from build123d import *

# Parameters (mm, degrees)
RESSALTO_EXTRUS_O1_DEPTH = 2
ESBO_O3_R                = 2
CORTE_EXTRUS_O2_DEPTH    = 10
ESBO_O5_R                = 1.65
CORTE_EXTRUS_O5_DEPTH    = 2


with BuildPart() as part:
    # Esboço1 → Ressalto-extrusão1 (new body)
    with BuildSketch(Plane(origin=(0, 0, 0), x_dir=(1, 0, 0), z_dir=(0, 1, 0))):
        Polygon((-114, 41.685), (-114, -79.875), (-51, -79.875), (0, -79.875), (0, 79.875), (-69.415, 79.875), align=None)
        Polygon((0, 79.875), (0, -79.875), (51.996049983, -79.875), (114, -79.875), (114, 41.685), (69.415, 79.875), align=None)
    extrude(amount=RESSALTO_EXTRUS_O1_DEPTH)

    # Esboço3 → Corte-extrusão2 (cut)
    with BuildSketch(Plane(origin=(0, 2, 0), x_dir=(1, 0, 0), z_dir=(0, 1, 0))):
        with Locations(Location((-45.14, -69.875, 0), (0, 0, 270))):
            Circle(ESBO_O3_R)
        with Locations(Location((45.14, -69.875, 0), (0, 0, 270))):
            Circle(ESBO_O3_R)
        with Locations(Location((-45.14, -49.875, 0), (0, 0, 270))):
            Circle(ESBO_O3_R)
        with Locations(Location((45.14, -49.875, 0), (0, 0, 270))):
            Circle(ESBO_O3_R)
    extrude(amount=-CORTE_EXTRUS_O2_DEPTH, mode=Mode.SUBTRACT)

    # Esboço5 → Corte-extrusão5 (cut)
    with BuildSketch(Plane(origin=(0, 2, 0), x_dir=(1, 0, 0), z_dir=(0, 1, 0))):
        with Locations(Location((100.5, 29.876998266, 0), (0, 0, 270))):
            Circle(ESBO_O5_R)
        with Locations(Location((100.5, 9.876998266, 0), (0, 0, 270))):
            Circle(ESBO_O5_R)
        with Locations(Location((-100.5, 29.876998266, 0), (0, 0, 270))):
            Circle(ESBO_O5_R)
        with Locations(Location((-100.5, 9.876998266, 0), (0, 0, 270))):
            Circle(ESBO_O5_R)
    extrude(amount=-CORTE_EXTRUS_O5_DEPTH, mode=Mode.SUBTRACT)


solid = part.part
CAD build for the part. Positions are in the model's coordinates, mm. Coordinates: 2 decimals unless noted, no trailing zeros. Loops run counter-clockwise (first coordinate to the right, second up) from the corner with the lowest first, then second, coordinate; pieces in that order, holes last. Notation, with made-up numbers: (-20, 31.5) - (28, 31.5) arc R35 ccw to (28, 63.5) - close; hole circle Ø3 at (23.5, -22.5). An arc over 180 degrees is marked (long way). Write item = value, one per line. Start each with the question number.
Q1. Cut at A-A, the plane y = 0.85. Give the number of separate pieces and of enclosed holes in the cut face, then the cut area to 3 significant figures.
Q2. Cut at B-B, the plane z = -57.5. List the corners of the cut face in (x, y).
Q3. Drill centre lines: L1, parallel to Z at x = -100.5, y = 1.65 (3 decimals); L2, parallel to X at y = 1.15, z = 48.5; L3, parallel to X at y = 0.95, z = -45.5. Where is each one in solid material? Low to high.
Q4. Cut at C-C, the plane x = -87. List the corners of the cut face in (y, z) (3 decimals).
Computed:
q1.separate_pieces = 1
q1.enclosed_holes = 8
q1.area = 34,600 mm²
q2.outline = (-95.54, 0) - (95.54, 0) - (95.54, 2) - (-95.54, 2) - close
q3.L1 = -53.249 to -31.527, -28.227 to -11.527, -8.227 to 79.875
q3.L2 = -114 to -46.59, -43.69 to 43.69, 46.59 to 114
q3.L3 = -109.55 to 109.55
q4.outline = (0, -64.812) - (2, -64.812) - (2, 79.875) - (0, 79.875) - close
